Source: three-view drawing plus pictorial views. Frame: mm from the lowest corner of the part. A direction names the side the tool comes from. Coordinates: 2 decimals unless noted, no trailing zeros. Write each loop counter-clockwise with the first axis right and the second up, starting at its lowest first coordinate (ties: lowest second). Pieces come first, ordered by that corner, then holes. Notation, with made-up numbers: (5.25, 22.5) - (49.25, 22.5) arc R25 cw to (49.25, 61.5) - close; hole circle Ø3 at (13.5, 50). An arc over 180 degrees is marked (long way). Put each result on its own line as item: value.
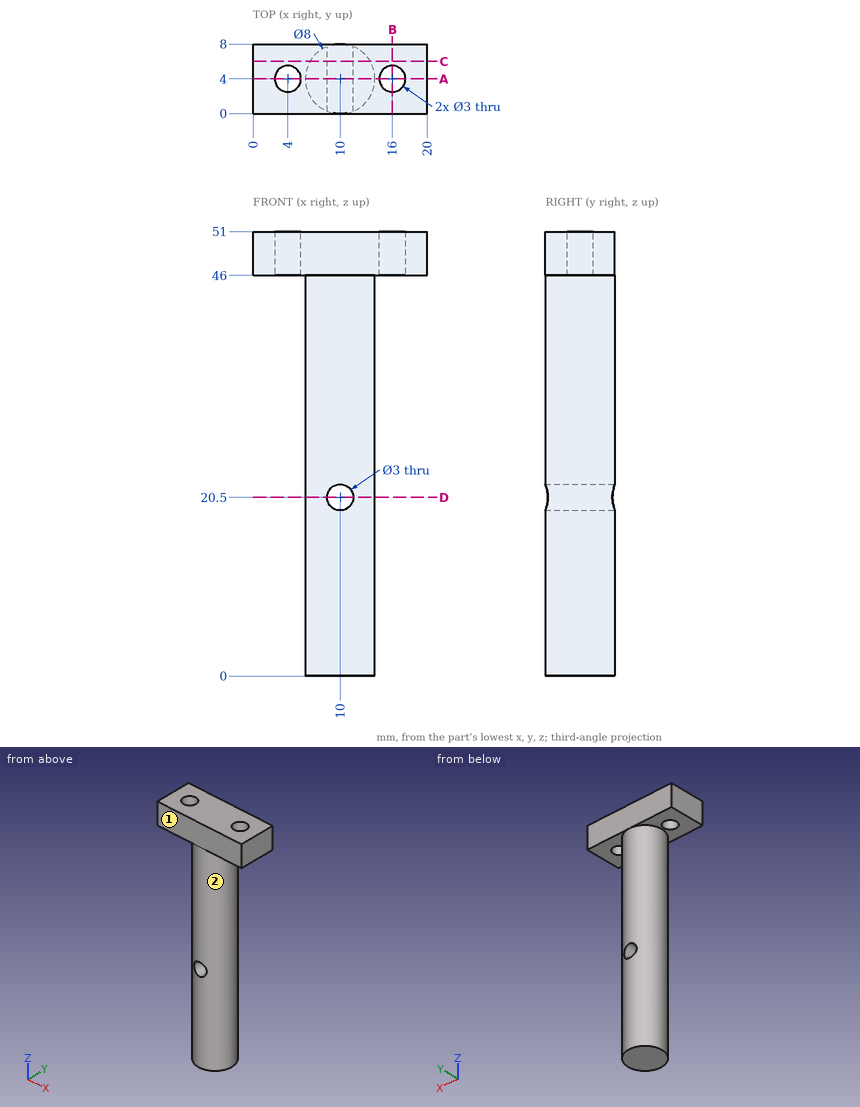
1. Section query D-D (z = 20.5). Return loops of the section in (x, y), then the cut area to 3 significant figures.
Answer below:
outline: (8.5, 0.29) - (8.5, 7.71) arc R4 ccw to start; (11.5, 0.29) arc R4 ccw to (11.5, 7.71) - close
area: 26.8 mm²
2. Section query C-C (y = 6). Return loops of the section in (x, z), then the cut area to 3 significant figures.
Answer below:
outline: (0, 46) - (6.54, 46) - (6.54, 0) - (13.46, 0) - (13.46, 46) - (20, 46) - (20, 51) - (0, 51) - close; hole circle Ø3 at (10, 20.5)
area: 412 mm²
3. Section query B-B (x = 16). Return loops of the section in (y, z), then the cut area to 3 significant figures.
Answer below:
outline: (0, 46) - (2.5, 46) - (2.5, 51) - (0, 51) - close; (5.5, 46) - (8, 46) - (8, 51) - (5.5, 51) - close
area: 25.0 mm²
4. Set-up query: the marked faces 1 and 2. Return all of +Z, -Z, +X, -X, +Y, -Y with unobstructed straight access to the full face (end or side cutting, diameter ignored); none if empty.
Answer below:
face 1: +Z, -Z, +X, -X, -Y
face 2: -Z
5. Ray query, probe 1 along Y at (x, z) = (16, 47.9); probe 2 along Z at (x, y) = (10, 5.5); probe 3 along Z at (x, y) = (3.5, 5.5). Return the intervals inside material, ascending. Write a range as from..to.
Answer below:
probe 1: y = 0..2.5, 5.5..8
probe 2: z = 0..19, 22..51
probe 3: z = 46..51
6. Pin query (flat end, axial travel): pin 1 Ø2 at (x, z) = (8.5, 39.5) entering from +Y; pin 2 Ø4 at (y, z) = (4.5, 40.5) entering from +X; pin 3 Ø3 at (x, z) = (5, 37.5) entering from +Y. Return the tip coordinate at first contact, or that it passes through.
Answer below:
pin 1: stops at y = 7.97
pin 2: stops at x = 14
pin 3: stops at y = 5.94
7. Section query A-A (y = 4). Return loops of the section in (x, z).
Answer below:
outline: (0, 46) - (2.5, 46) - (2.5, 51) - (0, 51) - close; (5.5, 46) - (6, 46) - (6, 0) - (14, 0) - (14, 46) - (14.5, 46) - (14.5, 51) - (5.5, 51) - close; (17.5, 46) - (20, 46) - (20, 51) - (17.5, 51) - close; hole circle Ø3 at (10, 20.5)
